Autodesk Inventor part; units mm, degrees
ref_plane "YZ Plane" through (0, 0, 0) normal (1, 0, 0) x (0, 1, 0)
ref_plane "XZ Plane" through (0, 0, 0) normal (0, 1, 0) x (-1, 0, 0)
ref_plane "XY Plane" through (0, 0, 0) normal (0, 0, 1) x (1, 0, 0)
sketch "Sketch1" plane through (0, 0, 0) normal (0, 1, 0) x (-1, 0, 0)
  line L0 (4.3002, 1.999) -> (5.4254, 0)
  line L1 (5.4254, 0) -> (11.9253, 0)
  line L2 (11.9253, 0) -> (13.4239, 1.5011)
  line L3 (13.4239, 1.5011) -> (13.4239, 9.4996)
  line L4 (13.4239, 9.4996) -> (11.9253, 11.0007)
  line L5 (11.9253, 11.0007) -> (5.4254, 11.0007)
  line L6 (5.4254, 11.0007) -> (4.3002, 8.9992)
  line L7 (4.3002, 8.9992) -> (0, 8.9992)
  line L8 (0, 8.9992) -> (0, 1.999)
  line L9 (0, 1.999) -> (4.3002, 1.999)
  line L10 (0, 8.9992) -> (4.3002, 8.9992)
  line L11 (4.3002, 8.9992) -> (5.4254, 11.0007)
  line L12 (5.4254, 11.0007) -> (11.9253, 11.0007)
  line L13 (11.9253, 11.0007) -> (13.4239, 9.4996)
  line L14 (13.4239, 9.4996) -> (13.4239, 1.5011)
  line L15 (13.4239, 1.5011) -> (11.9253, 0)
  line L16 (11.9253, 0) -> (5.4254, 0)
  line L17 (5.4254, 0) -> (4.3002, 1.999)
  line L18 (4.3002, 1.999) -> (0, 1.999)
  line L19 (0, 1.999) -> (0, 8.9992)
  point P0 (0, 0)
extrude "Extrusion1" add sketch "Sketch1" along normal blind 0.78
ref_plane "Work Plane1" through (-11.9253, 0, 5.5004) normal (0, 0, 1) x (1, 0, 0)
properties part number "32ch_ACF2TDT_board"
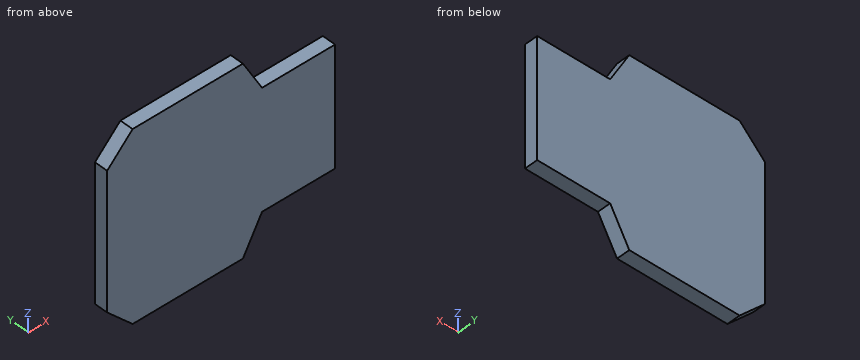
Build history of the part. All positions in model axes, mm. Coordinates: 2 decimals unless noted, no trailing zeros. Write each loop counter-clockwise with the first axis right and the second up, starting at its lowest first coordinate (ties: lowest second). Pieces come first, ordered by that corner, then holes.
(1) Cut at C-C on z = 10. List the corners of the cut face in (x, y), and give its area (3 significant figures).
(2) Drill centre lines: line 1 (Z direction, x = -0.75, y = 0.4); line 2 (Z direction, x = -13, y = 0.35); line 3 (X direction, y = 0.4, z = 1). Where is each one in solid material? Low to high.
(3) Cut at B-B on x = -3.5. List the corners of the cut face in (y, z), and give its area (3 significant figures).
(4) Cut at A-A on y = 0.4. List the corners of the cut face in (x, z), and give its area (3 significant figures).
Working result:
1. outline: (-12.92, 0) - (-4.86, 0) - (-4.86, 0.78) - (-12.92, 0.78) - close
1. area: 6.29 mm2
2. line 1: z = 2 to 9
2. line 2: z = 1.08 to 9.92
2. line 3: x = -12.92 to -4.86
3. outline: (0, 2) - (0.78, 2) - (0.78, 9) - (0, 9) - close
3. area: 5.46 mm2
4. outline: (-13.42, 1.5) - (-11.93, 0) - (-5.43, 0) - (-4.3, 2) - (0, 2) - (0, 9) - (-4.3, 9) - (-5.43, 11) - (-11.93, 11) - (-13.42, 9.5) - close
4. area: 126 mm2
